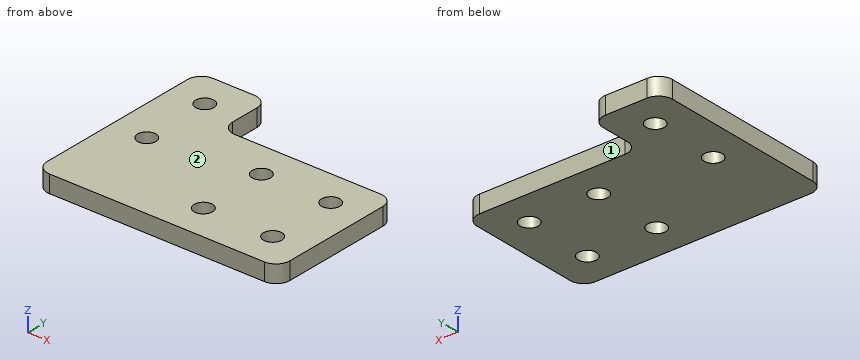
```python
from build123d import *

# Parameters (mm, degrees)
END_CAP_SKETCH_R        = 2.65
EXTRUDE_THICKNESS_DEPTH = 5


with BuildPart() as part:
    # End Cap Sketch → Extrude Thickness (new body)
    with BuildSketch(Plane.XY):
        with BuildLine():
            Line((-46, -20), (16, -20))
            ThreePointArc((16, -20), (18.828427125, -18.828427125), (20, -16))
            Line((20, -16), (20, 16))
            ThreePointArc((20, 16), (18.828427125, 18.828427125), (16, 20))
            Line((16, 20), (-26, 20))
            ThreePointArc((-26, 20), (-28.828427125, 21.171572875), (-30, 24))
            Line((-30, 24), (-30, 32.365))
            ThreePointArc((-30, 32.365), (-31.171572875, 35.193427125), (-34, 36.365))
            Line((-34, 36.365), (-46, 36.365))
            ThreePointArc((-46, 36.365), (-48.828427125, 35.193427125), (-50, 32.365))
            Line((-50, 32.365), (-50, -16))
            ThreePointArc((-50, -16), (-48.828427125, -18.828427125), (-46, -20))
        make_face()
        with Locations((-10, 10)):
            Circle(END_CAP_SKETCH_R, mode=Mode.SUBTRACT)
        with Locations((-10, -10)):
            Circle(END_CAP_SKETCH_R, mode=Mode.SUBTRACT)
        with Locations((10, 10)):
            Circle(END_CAP_SKETCH_R, mode=Mode.SUBTRACT)
        with Locations((10, -10)):
            Circle(END_CAP_SKETCH_R, mode=Mode.SUBTRACT)
        with Locations((-40, 26.365)):
            Circle(END_CAP_SKETCH_R, mode=Mode.SUBTRACT)
        with Locations((-40, 6.365)):
            Circle(END_CAP_SKETCH_R, mode=Mode.SUBTRACT)
    extrude(amount=EXTRUDE_THICKNESS_DEPTH)


solid = part.part
```
Design review of the part built by this model. Coordinates are the model's own, in mm. Face numbers are marked on the shaded views. A direction names the side the tool comes from. Give positions to 0.01 mm unless a question says otherwise; leave off trailing zeros. Order: outer loops, then holes, each group sorted by start corner. A loop starts at its lowest first (then second) coordinate and runs counter-clockwise, first axis right, second up. Notation, with made-up numbers: (86.25, 77) -> (145.25, 77) arc R16 cw to (145.25, 85) -> close; hole circle Ø9 at (62, -22). An arc over 180 degrees is marked (long way). Write item = value, one per line. Start each with the question number.
(1) For pin 1 (1.5 mm diameter, centred on y = 29, z = 1.5, fed in from +X); pin 2 (2.5 mm diameter, centred on x = -11, z = 2.5, fed in from +Y), all flat-tipped, find the tip position at first contact; note any pin that passes through.
(2) For the marked faces 1 and 2, list the 3-axis set-ups (+Z, -Z, +X, -X, +Y, -Y) from which the entire face can be reached by the end or side of a thin tool; tool diameter is ignored.
(3) To check wall thickness, follow line 1 along Y through (x, z) = (-10, 1); line 2 along Y through (x, z) = (-40, 2.15) (3 decimals); line 3 along X through (y, z) = (-9, 1.1). State the ranges of each line that lie inside material, in increasing order.
(4) We need section A-A on x = 10. Write out the cut boundary in (y, z).
(5) We need section D-D on x = -25. Write out the cut boundary in (y, z).
(6) We need section B-B on y = -10. Write out the cut boundary in (x, z).
(7) We need section C-C on z = 2.8. Write out the cut boundary in (x, y) (3 decimals), plus the area to 3 significant figures.
Numbers:
q1.pin_1 = -30
q1.pin_2 = 20
q2.face_1 = +Z, -Z, +X, +Y
q2.face_2 = +Z, +X, -X, +Y, -Y
q3.line_1 = -20 to -12.65, -7.35 to 7.35, 12.65 to 20
q3.line_2 = -20 to 3.715, 9.015 to 23.715, 29.015 to 36.365
q3.line_3 = -50 to -12.45, -7.55 to 7.55, 12.45 to 20
q4.outline = (-20, 0) -> (-12.65, 0) -> (-12.65, 5) -> (-20, 5) -> close; (-7.35, 0) -> (7.35, 0) -> (7.35, 5) -> (-7.35, 5) -> close; (12.65, 0) -> (20, 0) -> (20, 5) -> (12.65, 5) -> close
q5.outline = (-20, 0) -> (20, 0) -> (20, 5) -> (-20, 5) -> close
q6.outline = (-50, 0) -> (-12.65, 0) -> (-12.65, 5) -> (-50, 5) -> close; (-7.35, 0) -> (7.35, 0) -> (7.35, 5) -> (-7.35, 5) -> close; (12.65, 0) -> (20, 0) -> (20, 5) -> (12.65, 5) -> close
q7.outline = (-50, -16) arc R4 ccw to (-46, -20) -> (16, -20) arc R4 ccw to (20, -16) -> (20, 16) arc R4 ccw to (16, 20) -> (-26, 20) arc R4 cw to (-30, 24) -> (-30, 32.365) arc R4 ccw to (-34, 36.365) -> (-46, 36.365) arc R4 ccw to (-50, 32.365) -> close; hole circle Ø5.3 at (-40, 6.365); hole circle Ø5.3 at (-40, 26.365); hole circle Ø5.3 at (-10, -10); hole circle Ø5.3 at (-10, 10); hole circle Ø5.3 at (10, -10); hole circle Ø5.3 at (10, 10)
q7.area = 2,980 mm^2
